Part model, mm, in its own coordinate system. A direction names the side the tool comes from. Coordinates: 2 decimals unless noted, no trailing zeros. Write each loop counter-clockwise with the first axis right and the second up, starting at its lowest first coordinate (ties: lowest second). Pieces come first, ordered by that corner, then holes. Notation, with made-up numbers: (8, -7) - (32, -7) arc R23 cw to (32, 6) - close; hole circle Ø11 at (4, 21). An arc over 180 degrees is marked (long way). Write each question's results on one line, items separated by ' | '.
Autodesk Inventor part; units mm, degrees
ref_plane "YZ Plane" through (0, 0, 0) normal (1, 0, 0) x (0, 1, 0)
ref_plane "XZ Plane" through (0, 0, 0) normal (0, 1, 0) x (-1, 0, 0)
ref_plane "XY Plane" through (0, 0, 0) normal (0, 0, 1) x (1, 0, 0)
sketch "Sketch1" plane through (0, 0, 0) normal (1, 0, 0) x (0, 1, 0)
  line L0 (-0.7106, 0) -> (4.2636, 0)
  line L1 (0, 6.6675) -> (0, -6.6675)
  line L2 (2.54, -4.7625) -> (2.54, 4.7625)
  line L3 (2.54, 4.7625) -> (0, 4.7625)
  line L4 (0, 4.7625) -> (0, -4.7625)
  line L5 (0, -4.7625) -> (2.54, -4.7625)
  line L6 (2.54, -4.7625) -> (0, 4.7625) construction
  line L7 (2.54, 4.7625) -> (0, -4.7625) construction
  line L8 (0, 2.3495) -> (1.016, 2.3495)
  line L9 (1.016, 2.3495) -> (1.016, 4.7625)
  line L10 (0, -2.3495) -> (1.016, -2.3495)
  line L11 (1.016, -2.3495) -> (1.016, -4.7625)
  line L12 (1.27, 0) -> (3.553, 0) construction
  point P0 (0, 0)
  dimension "d0" = 9.525
  dimension "d1" = 2.54
  dimension "d2" = 0
  dimension "d3" = 1.016
  dimension "d4" = 4.699
  dimension "d5" = 2.413
  dimension "d6" = 2.413
extrude "Extrusion1" add sketch "Sketch1" along normal blind 9.906 contours L1 L8 L9 L3 L2 L0 | L0 L2 L5 L11 L10 L1
extrude "Extrusion2" add sketch "Sketch1" against normal blind 12.573
sketch "Sketch2" plane through (0, 0, 0) normal (0, 1, 0) x (-1, 0, 0)
  line L0 (-1.3208, 0) -> (7.9248, 0)
  line L1 (0, -4.445) -> (0, 4.445)
  point P0 (0, 0)
  point P1 (3.429, 0)
  dimension "d11" = 3.429
hole "Hole1" at (-3.429, 0, 0) direction (0, 1, 0) diameter 4.7625 end through all counterbore diameter 6.223 counterbore depth 1.016
sketch "Sketch3" plane through (9.906, 0, -2.3495) normal (0, -1, 0) x (1, 0, 0)
  line L0 (-22.479, 5.715) -> (-17.399, 5.715)
  line L1 (-17.399, 5.715) -> (-17.399, -1.016)
  line L2 (-17.399, -1.016) -> (-22.479, -1.016)
  line L3 (-22.479, -1.016) -> (-22.479, 5.715)
  line L4 (-34.3558, 2.3495) -> (5.726, 2.3495)
  line L5 (-9.906, 9.0932) -> (-9.906, -4.3307)
  line L6 (-9.906, 2.3495) -> (-28.6298, 2.3495) construction
  line L7 (-22.479, 7.112) -> (0, 7.112)
  line L8 (-22.479, 5.715) -> (-11.684, 5.715)
  line L9 (-11.684, 5.715) -> (-11.684, 7.112)
  line L10 (-11.684, 7.112) -> (-22.479, 7.112)
  line L11 (-22.479, 7.112) -> (-22.479, 5.715)
  line L12 (0, -2.413) -> (-22.479, -2.413)
  line L13 (-22.479, -1.016) -> (-11.684, -1.016)
  line L14 (-11.684, -1.016) -> (-11.684, -2.413)
  line L15 (-11.684, -2.413) -> (-22.479, -2.413)
  line L16 (-22.479, -2.413) -> (-22.479, -1.016)
  dimension "d22" = 5.08
  dimension "d30" = 6.731
  dimension "d45" = 10.795
  dimension "d46" = 10.795
extrude "Extrusion3" add sketch "Sketch3" along normal blind 0.889 contours L11 L7 L9 L8 L0 | L0 L1 L4 L3 | L4 L1 L2 L3 | L2 L13 L14 L12 L16
chamfer "Chamfer2" distance 0.254 angle 45 2 edges at (-1.778, -0.889, 4.064) (-1.778, -0.889, -4.064)
fillet "Fillet1" radius 0.7937 4 edges at (9.906, 0.508, 2.3495) (9.906, 0.508, -2.3495) (9.906, 1.778, 4.7625) (9.906, 1.778, -4.7625)
fillet "Fillet2" radius 0.381 2 edges at (0, 0.508, -4.7625) (0, 0.508, 4.7625)
sketch "Sketch4" plane through (0, 0, 0) normal (0, 1, 0) x (-1, 0, 0)
  circle A0 centre (3.429, 0) radius 2.3813
  circle A1 centre (3.429, 0) radius 3.175
  point P0 (0, 0)
  dimension "d34" = 6.35
sketch "Sketch5" plane through (9.906, -0.889, -2.3495) normal (0, -1, 0) x (1, 0, 0)
  line L0 (-26.9748, 2.3495) -> (4.4958, 2.3495)
  line L1 (-9.906, 9.017) -> (-9.906, -4.318)
  line L2 (-22.479, 7.112) -> (-22.479, -2.413)
  line L3 (-20.955, -1.143) -> (-22.479, -1.143)
  line L4 (-22.479, -1.143) -> (-22.479, 5.842)
  line L5 (-22.479, 5.842) -> (-20.955, 5.842)
  line L6 (-20.955, 5.842) -> (-20.955, -1.143)
  line L7 (-20.955, -1.143) -> (-22.479, 5.842) construction
  line L8 (-22.479, -1.143) -> (-20.955, 5.842) construction
  point P0 (-9.906, 2.3495)
  point P1 (-21.717, 2.3495)
  dimension "d47" = 6.985
  dimension "d48" = 1.524
extrude "Extrusion4" add sketch "Sketch5" along normal blind 0.3048
chamfer "Chamfer4" distance 1.27 distance2 1.905 1 edges at (-12.573, 0.8255, -4.7625) measured on face at (-12.573, 1.397, -1.1642)
chamfer "Chamfer5" distance 1.905 distance2 1.27 1 edges at (-12.573, 0.8255, 4.7625) measured on face at (-9.0593, 0.254, 4.7625)
fillet "Fillet4" radius 0.7937 2 edges at (-12.573, -1.0414, -3.4925) (-12.573, -1.0414, 3.4925)
fillet "Fillet5" radius 0.7937 4 edges at (-12.573, 0.8255, 3.4925) (-10.668, 0.8255, 4.7625) (-12.573, 0.8255, -3.4925) (-10.668, 0.8255, -4.7625)
fillet "Fillet6" radius 1.651 4 edges at (0, 0.508, -2.3495) (0, 0.508, 2.3495) (-7.493, -0.4445, 3.3655) (-7.493, -0.4445, -3.3655)
sketch "Sketch6" plane through (0, 0, 0) normal (0, 0, 1) x (1, 0, 0)
  line L0 (-11.049, -1.1938) -> (-11.7793, -1.1938)
  line L1 (-11.049, -0.889) -> (-11.049, -1.1938)
  line L2 (-2.032, -0.889) -> (-10.4277, -0.889)
  line L3 (-11.049, -1.1938) -> (-2.032, -0.889)
  point P0 (0, 0)
  dimension "d51" = 1.936
properties part number "J005044" material "STAINLESS STEEL, 303"
(1) Wall check: line 1 (X direction, y = 0.35, z = 0); line 2 (X direction, y = 2.2, z = 0); line 3 (Z direction, x = -3, y = 1.15). Give the ranges that are in metal, low to high. Write a range as from..to.
Return value:
line 1: x = -12.57..-6.54, -0.32..9.91 | line 2: x = -12.57..-5.81, -1.05..9.91 | line 3: z = -4.76..-2.34, 2.34..4.76
(2) Saw through at B-B on x = 3. Write the cut outline in (y, z), then the cut area to 3 significant figures.
Return value:
outline: (0, -2.35) - (1.02, -2.35) - (1.02, -4.76) - (2.54, -4.76) - (2.54, 4.76) - (1.02, 4.76) - (1.02, 2.35) - (0, 2.35) - close | area: 19.3 mm^2
(3) Flat gauge pins, fed straight in: P1, Ø0.7, axis at y = -0.5, z = -4, coming from the +X side; P2, Ø0.8, axis at x = 5.5, y = 0.5, coming from the +Z side; P3, Ø3, axis at x = -4, z = -1, coming from the -Y side. Where does each tip first touch, or does it go through?
Return value:
P1: stops at x = -1.78 | P2: stops at z = 2.35 | P3: stops at y = 1.02
(4) Saw through at A-A on z = 0. Write the cut outline in (x, y).
Return value:
outline: (-12.57, -1.19) - (-11.05, -1.19) - (-11.05, -0.89) - (-7.49, -0.89) - (-7.49, 0) - (-6.54, 0) - (-6.54, 1.02) - (-5.81, 1.02) - (-5.81, 2.54) - (-12.57, 2.54) - close; (-1.05, 1.02) - (-0.32, 1.02) - (-0.32, 0) - (9.91, 0) - (9.91, 2.54) - (-1.05, 2.54) - close
(5) Saw through at D-D on y = -0.3. Write the cut outline in (x, z).
Return value:
outline: (-12.57, -3.07) arc R0.79 ccw to (-12.22, -3.73) - (-10.87, -4.63) arc R0.79 ccw to (-10.43, -4.76) - (-1.78, -4.76) - (-1.78, -3.37) - (-5.84, -3.37) arc R1.65 cw to (-7.49, -1.71) - (-7.49, 1.71) arc R1.65 cw to (-5.84, 3.37) - (-1.78, 3.37) - (-1.78, 4.76) - (-10.43, 4.76) arc R0.79 ccw to (-10.87, 4.63) - (-12.22, 3.73) arc R0.79 ccw to (-12.57, 3.07) - close
(6) Saw through at C-C on y = 0.6. Write the cut outline in (x, z), then the cut area to 3 significant figures.
Return value:
outline: (-12.57, -3.07) arc R0.79 ccw to (-12.22, -3.73) - (-10.87, -4.63) arc R0.79 ccw to (-10.43, -4.76) - (-0.38, -4.76) arc R0.38 ccw to (0, -4.38) - (0, -4) arc R1.65 cw to (1.65, -2.35) - (9.11, -2.35) arc R0.79 ccw to (9.91, -1.56) - (9.91, 1.56) arc R0.79 ccw to (9.11, 2.35) - (1.65, 2.35) arc R1.65 cw to (0, 4) - (0, 4.38) arc R0.38 ccw to (-0.38, 4.76) - (-10.43, 4.76) arc R0.79 ccw to (-10.87, 4.63) - (-12.22, 3.73) arc R0.79 ccw to (-12.57, 3.07) - close; hole circle Ø6.22 at (-3.43, 0) | area: 134 mm^2
(7) 3-axis set-ups, long thin cutter, end or side, ignore diameter. For faces 1 (the cylindrical face through (0.496, 0.515, 2.82)), 2 (the flat face through (-3.8, -0.4, 3.366)), 3 (the flat face through (5, 1.016, -3)): which of +Z, -Z, +X, -X, +Y, -Y reach the whole face in a straight line?
Return value:
face 1: +Z, +X, -Y | face 2: +X, -Y | face 3: -Z, +X, -Y
(8) Two-plate mould, pull along Z, no slides. Class faces 4 (the flat face through (-9, -0.889, 0)), 5 (the cylindrical face through (0.471, 0.515, -2.846)), 6 (the flat face through (-3.8, -0.4, -3.366)): released by +Z, released by -Z, zero draft, split by the parting line, or undercut.
Return value:
face 4: zero draft | face 5: released by -Z | face 6: undercut
